from build123d import *

# Parameters (mm, degrees)
F0_W     = 9
F0_H     = 8
F0_R     = 17
F1_DEPTH = 38
F2_W     = 20
F2_H     = 14
F3_DEPTH = 113.538
F5_W     = 18
F5_H     = 20
F6_DEPTH = 71.628


with BuildPart() as f1:
    # F0 (on Front) → F1 (new body)
    with BuildSketch(Plane.XZ):
        with BuildLine():
            ThreePointArc((-20.1246117975, -18), (-27, 0), (-20.1246117975, 18))
            Line((-20.1246117975, 18), (-44, 18))
            Line((-44, 18), (-44, -18))
            Line((-44, -18), (-20.1246117975, -18))
        make_face()
        with Locations((-35.5, 0)):
            Rectangle(F0_W, F0_H, mode=Mode.SUBTRACT)
        with BuildLine():
            ThreePointArc((20.1246117975, -18), (25.222653692, -9.6341964239), (27, 0))
            ThreePointArc((27, 0), (25.222653692, 9.6341964239), (20.1246117975, 18))
            Line((20.1246117975, 18), (-20.1246117975, 18))
            ThreePointArc((-20.1246117975, 18), (-27, 0), (-20.1246117975, -18))
            Line((-20.1246117975, -18), (20.1246117975, -18))
        make_face()
        Circle(F0_R, mode=Mode.SUBTRACT)
        with BuildLine():
            Line((-20.1246117975, 18), (20.1246117975, 18))
            ThreePointArc((20.1246117975, 18), (0, 27), (-20.1246117975, 18))
        make_face()
        with BuildLine():
            ThreePointArc((20.1246117975, 18), (25.222653692, 9.6341964239), (27, 0))
            ThreePointArc((27, 0), (25.222653692, -9.6341964239), (20.1246117975, -18))
            Line((20.1246117975, -18), (44, -18))
            Line((44, -18), (44, 18))
            Line((44, 18), (20.1246117975, 18))
        make_face()
        with Locations((36.5, 0)):
            Rectangle(F0_W, F0_H, mode=Mode.SUBTRACT)
        with BuildLine():
            ThreePointArc((-20.1246117975, -18), (0, -27), (20.1246117975, -18))
            Line((20.1246117975, -18), (-20.1246117975, -18))
        make_face()
    extrude(amount=F1_DEPTH)

    # F2 (on face) → F3 (cut)
    with BuildSketch(Plane(origin=(-44, 0, 0), x_dir=(0, -1, 0), z_dir=(-1, 0, 0))):
        with Locations((19, 0)):
            Rectangle(F2_W, F2_H)
    extrude(amount=-F3_DEPTH, mode=Mode.SUBTRACT)

    # F5 (on offset) → F6 (cut)
    with BuildSketch(Plane.XY.offset(27)):
        with Locations((0, -19)):
            Rectangle(F5_W, F5_H)
    extrude(amount=-F6_DEPTH, mode=Mode.SUBTRACT)


solid = f1.part
Verification items for the finished model (mm, model axes). A direction names the side the tool comes from. Coordinates: 2 decimals unless noted, no trailing zeros. Order: outer loops, then holes, each group sorted by start corner. A loop starts at its lowest first (then second) coordinate and runs counter-clockwise, first axis right, second up.
Item 1: Access from +Z, -Z, +X, -X, +Y, -Y to the whole of each face (thin tool, end or side, straight path). Record for faces 5 (the face through (-31, -4, 0)), 6 (the face through (32, -19, -18)), 7 (the face through (-30, -9, 0)), 8 (the face through (-9, -19, -20)).
Filled in:
face 5: +Y, -Y
face 6: -Z, +X, +Y, -Y
face 7: +X, -X
face 8: +Z, -Z
Item 2: Release check for a two-part mould opening along X. For faces 1 (the face through (-44, -19, 8)), 2 (the face through (-30, -29, 0)), 3 (the face through (0, -29, -22)), 4 (the face through (-9.56, -18.73, 25.25)) record: +X half, -X half, draft (parallel to the pull), parting line (faces both ways), or undercut.
Filled in:
face 1: -X half
face 2: draft
face 3: undercut
face 4: parting line
Item 3: Material ranges on L1, parallel to Z at x = 30.5, y = -23; L2, parallel to X at y = -10.5, z = -17.5; L3, parallel to X at y = -7, z = -3.5, recorded low to high.
Filled in:
L1: z = -18 to -7, 7 to 18
L2: x = -44 to -9, 9 to 44
L3: x = -44 to -40, -31 to -16.64, 16.64 to 32, 41 to 44
Item 4: Section check A-A, the plane x = -36. Enter the section's corners in (y, z), then the cut area to 3 significant figures.
Filled in:
outline: (-38, -18) - (0, -18) - (0, -4) - (-9, -4) - (-9, -7) - (-29, -7) - (-29, -4) - (-38, -4) - close; (-38, 4) - (-29, 4) - (-29, 7) - (-9, 7) - (-9, 4) - (0, 4) - (0, 18) - (-38, 18) - close
area: 944 mm2
Item 5: Section check B-B, the plane y = -12. Enter the section's corners in (x, z).
Filled in:
outline: (-44, -18) - (-20.12, -18) arc R27 ccw to (-9, -25.46) - (-9, -14.42) arc R17 cw to (-15.49, -7) - (-44, -7) - close; (-44, 7) - (-15.49, 7) arc R17 cw to (-9, 14.42) - (-9, 25.46) arc R27 ccw to (-20.12, 18) - (-44, 18) - close; (9, -25.46) arc R27 ccw to (20.12, -18) - (44, -18) - (44, -7) - (15.49, -7) arc R17 cw to (9, -14.42) - close; (9, 14.42) arc R17 cw to (15.49, 7) - (44, 7) - (44, 18) - (20.12, 18) arc R27 ccw to (9, 25.46) - close
Item 6: Section check C-C, the plane z = 0. Give the number of separate pieces and of enclosed holes in the cut face, then the cut area to 3 significant figures.
Filled in:
separate pieces: 8
enclosed holes: 0
area: 648 mm2
Item 7: Depth check by flat-ended pin: pin 1 (12 mm diameter, centred on x = -13.5, z = 12.5, fed in from +Y); pin 2 (4.5 mm diameter, centred on x = 37, y = -4, fed in from -Z); pin 3 (2 mm diameter, centred on x = 16, y = -8, fed in from +Z); pin 4 (2 mm diameter, centred on x = 12, y = -17.5, fed in from -Z). Enter the tip coordinate at first touch or a pass-through.
Filled in:
pin 1: stops at y = 0
pin 2: stops at z = -18
pin 3: stops at z = 22.45
pin 4: stops at z = -24.66
Item 8: Section check D-D, the plane x = 25. Enter the section's corners in (y, z), then the cut area to 3 significant figures.
Filled in:
outline: (-38, -18) - (0, -18) - (0, 18) - (-38, 18) - close; hole (-29, -7) - (-9, -7) - (-9, 7) - (-29, 7) - close
area: 1,090 mm2
